Geometry: see drawing. Coordinates: mm, zero at the bounding-box minimum. Coordinates: 2 decimals unless noted, no trailing zeros. Order: outer loops, then holes, each group sorted by start corner. A loop starts at its lowest first (then second) coordinate and runs counter-clockwise, first axis right, second up. Notation, with made-up numbers: M -8,56.5 L 44,56.5 A23 cw 44,88.5 Z; hole C 67,59 d7. An arc over 180 degrees is marked long. Answer in a Markdown table with one row per item.
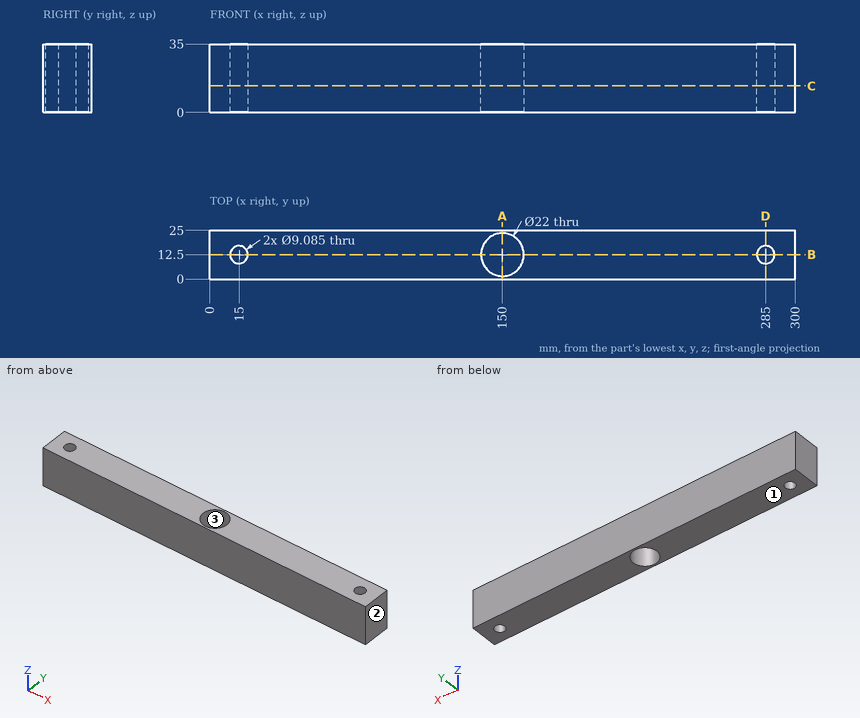
1) Cut plane B-B, the plane y = 12.5. Output: boundary loops of the cut face in (x, z), and give its area (3 significant figures).
Resolved:
| item | result |
|---|---|
| outline | M 0,0 L 10.46,0 L 10.46,35 L 0,35 Z; M 19.54,0 L 139,0 L 139,35 L 19.54,35 Z; M 161,0 L 280.46,0 L 280.46,35 L 161,35 Z; M 289.54,0 L 300,0 L 300,35 L 289.54,35 Z |
| area | 9,090 mm2 |
2) Cut plane C-C, the plane z = 13.5. Output: boundary loops of the cut face in (x, y) (1 decimal), and give its area (3 significant figures).
Resolved:
| item | result |
|---|---|
| outline | M 0,0 L 300,0 L 300,25 L 0,25 Z; hole C 15,12.5 d9.1; hole C 150,12.5 d22; hole C 285,12.5 d9.1 |
| area | 6,990 mm2 |
3) Material intervals for probe 1 along Y at (x, z) = (285, 28); probe 2 along X at (y, z) = (9, 19) (1 decimal); probe 3 along X at (y, z) = (18, 6), sorted ascending.
Resolved:
| item | result |
|---|---|
| probe 1 | y = 0 to 7.96, 17.04 to 25 |
| probe 2 | x = 0 to 12.1, 17.9 to 139.6, 160.4 to 282.1, 287.9 to 300 |
| probe 3 | x = 0 to 140.47, 159.53 to 300 |
4) Cut plane D-D, the plane x = 285. Output: boundary loops of the cut face in (y, z).
Resolved:
| item | result |
|---|---|
| outline | M 0,0 L 7.96,0 L 7.96,35 L 0,35 Z; M 17.04,0 L 25,0 L 25,35 L 17.04,35 Z |
5) Contact query for a flat-ended pin moving along its axis: pin 1 (8 mm diameter, centred on x = 155, y = 16, fed in from -Z). Output: stop coordinate, or through.
Resolved:
| item | result |
|---|---|
| pin 1 | passes through |
6) Cut plane A-A, the plane x = 150. Output: boundary loops of the cut face in (y, z).
Resolved:
| item | result |
|---|---|
| outline | M 0,0 L 1.5,0 L 1.5,35 L 0,35 Z; M 23.5,0 L 25,0 L 25,35 L 23.5,35 Z |
7) Mould query, pull axis X, two halves, no side actions, for the marked faces 1, 2 and 3. Classes: +X half, -X half, draft (parallel to the pull), parting line (faces both ways), or undercut.
Resolved:
| item | result |
|---|---|
| face 1 | draft |
| face 2 | +X half |
| face 3 | undercut |
